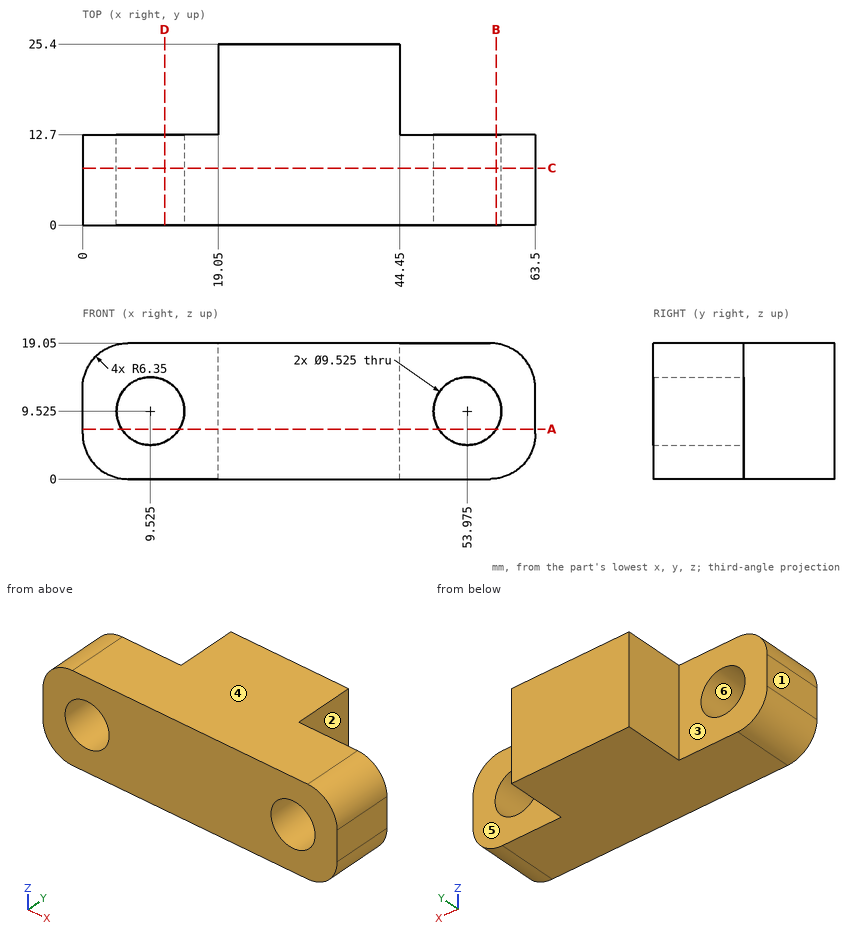
Design review of the part shown in the three views and the two pictorial views. Dimensions are in mm from the part's minimum x, y and z. A direction names the side the tool comes from. Round coordinates to 2 decimals unless told otherwise and drop trailing zeros. Write each loop counter-clockwise with the first axis right and the second up, starting at its lowest first coordinate (ties: lowest second). Pieces come first, ordered by that corner, then holes. Notation, with made-up numbers: (25, -4.75) -> (72, -4.75) arc R19 cw to (72, 1.25) -> close; hole circle Ø2 at (7.5, 66.5). An arc over 180 degrees is marked (long way). Use one line per item in the form item = value.
1) To check wall thickness, follow L1, parallel to X at y = 4, z = 9.5; L2, parallel to X at y = 8, z = 8.25; L3, parallel to X at y = 20.25, z = 8.75. State the ranges of each line that lie inside material, in increasing order. Write a range as from..to.
Found:
L1 = 0..4.76, 14.29..49.21, 58.74..63.5
L2 = 0..4.94, 14.11..49.39, 58.56..63.5
L3 = 19.05..44.45
2) Mouldability with a two-part tool opening along Z and no side actions: class the marked faces 4, 5 and 6 as +Z half, -Z half, draft (parallel to the pull), parting line (faces both ways), or undercut.
Found:
face_4 = +Z half
face_5 = draft
face_6 = undercut
3) Take a section at A-A, the plane z = 7. Write out the cut boundary in (x, y).
Found:
outline = (0, 0) -> (5.49, 0) -> (5.49, 12.7) -> (0, 12.7) -> close; (13.56, 0) -> (49.94, 0) -> (49.94, 12.7) -> (44.45, 12.7) -> (44.45, 25.4) -> (19.05, 25.4) -> (19.05, 12.7) -> (13.56, 12.7) -> close; (58.01, 0) -> (63.5, 0) -> (63.5, 12.7) -> (58.01, 12.7) -> close
4) Take a section at C-C, the plane y = 8. Count the separate pieces of the cut face and the enclosed holes in it, and give its area (3 significant figures).
Found:
separate_pieces = 1
enclosed_holes = 2
area = 1,030 mm2
5) Clearance check with flat-ended pins moving along their axes: pin 1 (6 mm diameter, centred on y = 22, z = 9.5, fed in from +X); pin 2 (11 mm diameter, centred on x = 9.525, z = 9.525, fed in from -Y); pin 3 (9.5 mm diameter, centred on x = 7, z = 6.5, fed in from +Y). State where each tip first meets the part, or that it passes through.
Found:
pin_1 = 44.45
pin_2 = 0
pin_3 = 12.7
6) Take a section at D-D, the plane x = 11.5. Write out the cut boundary in (y, z).
Found:
outline = (0, 0) -> (12.7, 0) -> (12.7, 5.19) -> (0, 5.19) -> close; (0, 13.86) -> (12.7, 13.86) -> (12.7, 19.05) -> (0, 19.05) -> close
7) Take a section at B-B, the plane x = 58. Write out the cut boundary in (y, z).
Found:
outline = (0, 0.06) -> (12.7, 0.06) -> (12.7, 6.98) -> (0, 6.98) -> close; (0, 12.07) -> (12.7, 12.07) -> (12.7, 18.99) -> (0, 18.99) -> close
8) Tool access review of the marked faces 1, 2 and 3: name each direction out of +Z, -Z, +X, -X, +Y, -Y from which nothing blocks a thin tool from reaching the whole face with its end or side.
Found:
face_1 = +Z, -Z, -X, +Y, -Y
face_2 = +Z, -Z, +X, +Y
face_3 = +Z, -Z, -X, +Y
